Build history of the part. All positions in model axes, mm. A direction names the side the tool comes from. Round coordinates to 2 decimals unless told otherwise and drop trailing zeros. Write each loop counter-clockwise with the first axis right and the second up, starting at its lowest first coordinate (ties: lowest second). Pieces come first, ordered by that corner, then holes. Notation, with made-up numbers: (54, -0.75) - (94, -0.75) arc R15 cw to (94, 5.25) - close; hole circle Ø2 at (73.25, 6.25). An arc over 180 degrees is marked (long way). Answer as a JSON object with one key per item and string values. Group by question number.
Item 1: Slice it at D-D, the plane y = 112.5. List the corners of the cut face in (x, z), then the cut area to 3 significant figures.
Item 2: Slice it at C-C, the plane x = 0. Give the number of separate pieces and of enclosed holes in the cut face, then the cut area to 3 significant figures.
Item 3: Two-plate mould, pull along Z, no slides. Class faces 1 (the cylindrical face through (159.517, 16.224, 106.685)), 2 (the cylindrical face through (1.1, 16.22, -261.29)), 3 (the flat face through (158, 193, 91)), 4 (the cylindrical face through (-205.935, 208.776, 100.557)): +Z half, -Z half, draft (parallel to the pull), parting line (faces both ways), or undercut.
Item 4: Flat gauge pins, fed straight in: pin 1 (1.5 mm diameter, centred on y = 72.5, z = 44, fed in from -X); pin 2 (8 mm diameter, centred on y = 115, z = 98, fed in from +X); pin 3 (12 mm diameter, centred on x = 64.5, y = 72.5, fed in from +Z). Where does each tip first touch, or does it go through?
Item 5: Slice it at A-A, the plane z = -156. List the corners of the cut face in (x, y), then the cut area to 3 significant figures.
Item 6: Probe line 1 (X direction, y = 112, z = 120); line 2 (Z direction, x = 52, y = 96.5); line 3 (Z direction, x = -204, y = 197.5). List the from-to ranges inside material, lowest first. Write a range as from..to.
Item 7: Which spindle directions (+Z, -Z, +X, -X, +Y, -Y) get a long thin tool onto all of the face, cutting with end or side? Do faces 5 (the flat face through (122.633, 16.224, 128.537)), 6 (the cylindrical face through (94.619, 110.925, -103.186)), 7 (the cylindrical face through (55.179, 83.646, 152.605)). Say none if no direction does.
Item 8: Slice it at B-B, the plane y = 74.5. List the corners of the cut face in (x, z), then the cut area to 3 significant figures.
from build123d import *

# Parameters (mm, degrees)
SKETCH1_R                = 140
SKETCH1_R_2              = 97
BOSS_EXTRUDE3_DEPTH      = 225
BOSS_EXTRUDE4_START      = -32
SKETCH4_R                = 23.5
BOSS_EXTRUDE4_DEPTH      = 32
CIRPATTERN2_COUNT        = 3
MIRROR1_START            = -32
MIRROR1_COPY_1_SKETCH_R  = 23.5
MIRROR1_COPY_1_DEPTH     = 32
MIRROR1_COPY_2_SKETCH_R  = 23.5
MIRROR1_COPY_2_DEPTH     = 32
BOSS_EXTRUDE5_REACH      = 533.421
BOSS_EXTRUDE5_END_RADIUS = 140
SKETCH6_R                = 100
SKETCH7_R                = 50
CUT_EXTRUDE1_DEPTH       = 25
SKETCH8_R                = 28
CUT_EXTRUDE2_DEPTH       = 512.827938218
SKETCH9_R                = 12
CUT_EXTRUDE3_DEPTH       = 15
CIRPATTERN3_COUNT        = 3


with BuildPart() as part:
    # Sketch1 → Boss-Extrude3 (new body)
    with BuildSketch(Plane(origin=(0, 0, 0), x_dir=(1, 0, 0), z_dir=(0, 1, 0))):
        with Locations(Location((0, 0, 0), (0, 0, 270))):
            Circle(SKETCH1_R)
        with Locations(Location((0, 0, 0), (0, 0, 270))):
            Circle(SKETCH1_R_2, mode=Mode.SUBTRACT)
    extrude(amount=BOSS_EXTRUDE3_DEPTH)

    # Sketch4 → Boss-Extrude4 (add)
    with BuildSketch(Plane(origin=(0, 225, 0), x_dir=(1, 0, 0), z_dir=(0, 1, 0)).offset(BOSS_EXTRUDE4_START)):
        with BuildLine():
            ThreePointArc((50, 211.303564756), (0, 261.303564756), (-50, 211.303564756))
            Line((-50, 211.303564756), (-50, 130.766968306))
            ThreePointArc((-50, 130.766968306), (0, 140), (50, 130.766968306))
            Line((50, 130.766968306), (50, 211.303564756))
        make_face()
        with Locations(Location((0, 211.303564756, 0), (0, 0, 270))):
            Circle(SKETCH4_R, mode=Mode.SUBTRACT)
    boss_extrude4 = extrude(amount=BOSS_EXTRUDE4_DEPTH)

    # CirPattern2: Boss-Extrude4 ×3 about axis
    cirpattern2_axis = Axis((0, 0, 0), (0, 1, 0))
    for i in range(1, CIRPATTERN2_COUNT):
        add(boss_extrude4.rotate(cirpattern2_axis, i * 360 / CIRPATTERN2_COUNT))

    # Mirror1: Boss-Extrude4 across plane
    add(boss_extrude4.mirror(Plane.ZX.offset(112.5)))

    # Mirror1 copy 1 sketch → Mirror1 copy 1 (add)
    with BuildSketch(Plane(origin=(0, 0, 0), x_dir=(-0.4999999999999998, 0, -0.8660254037844387), z_dir=(0, -1, 0)).offset(MIRROR1_START)):
        with BuildLine():
            ThreePointArc((50, -211.303564756), (0, -261.303564756), (-50, -211.303564756))
            Line((-50, -211.303564756), (-50, -130.766968306))
            ThreePointArc((-50, -130.766968306), (0, -140), (50, -130.766968306))
            Line((50, -130.766968306), (50, -211.303564756))
        make_face()
        with Locations((0, -211.303564756)):
            Circle(MIRROR1_COPY_1_SKETCH_R, mode=Mode.SUBTRACT)
    extrude(amount=MIRROR1_COPY_1_DEPTH)

    # Mirror1 copy 2 sketch → Mirror1 copy 2 (add)
    with BuildSketch(Plane(origin=(0, 0, 0), x_dir=(-0.5000000000000004, 0, 0.8660254037844384), z_dir=(0, -1, 0)).offset(MIRROR1_START)):
        with BuildLine():
            ThreePointArc((50, -211.303564756), (0, -261.303564756), (-50, -211.303564756))
            Line((-50, -211.303564756), (-50, -130.766968306))
            ThreePointArc((-50, -130.766968306), (0, -140), (50, -130.766968306))
            Line((50, -130.766968306), (50, -211.303564756))
        make_face()
        with Locations((0, -211.303564756)):
            Circle(MIRROR1_COPY_2_SKETCH_R, mode=Mode.SUBTRACT)
    extrude(amount=MIRROR1_COPY_2_DEPTH)

    # Boss-Extrude5: up to this cylinder (the profile starts outside it)
    boss_extrude5_end = Plane(origin=(0, 112.5, 0), z_dir=(0, -1, 0)) * Cylinder(BOSS_EXTRUDE5_END_RADIUS, 1347.842, mode=Mode.PRIVATE)
    # Sketch6 → Boss-Extrude5 (add, up to the surface)
    with BuildSketch(Plane.XY.offset(160), mode=Mode.PRIVATE) as boss_extrude5_sk1:
        with Locations((0, 112.5)):
            Circle(SKETCH6_R)
    boss_extrude5_tool1 = extrude(boss_extrude5_sk1.sketch, amount=-BOSS_EXTRUDE5_REACH, mode=Mode.PRIVATE) - boss_extrude5_end
    add(boss_extrude5_tool1.solids().sort_by_distance((0, 112.5, 160))[0])

    # Sketch7 → Cut-Extrude1 (cut)
    with BuildSketch(Plane.XY.offset(160)):
        with Locations((0, 112.5)):
            Circle(SKETCH7_R)
    extrude(amount=-CUT_EXTRUDE1_DEPTH, mode=Mode.SUBTRACT)

    # Sketch8 → Cut-Extrude2 (cut, through all)
    with BuildSketch(Plane.XY.offset(135)):
        with Locations((0, 112.5)):
            Circle(SKETCH8_R)
    extrude(amount=-CUT_EXTRUDE2_DEPTH, mode=Mode.SUBTRACT)

    # Sketch9 → Cut-Extrude3 (cut)
    with BuildSketch(Plane.XY.offset(160)):
        with Locations((0, 186.428214738)):
            Circle(SKETCH9_R)
    cut_extrude3 = extrude(amount=-CUT_EXTRUDE3_DEPTH, mode=Mode.SUBTRACT)

    # CirPattern3: Cut-Extrude3 ×3 about axis
    cirpattern3_axis = Axis((0, 112.5, 0), (0, 0, 1))
    for i in range(1, CIRPATTERN3_COUNT):
        add(cut_extrude3.rotate(cirpattern3_axis, i * 360 / CIRPATTERN3_COUNT), mode=Mode.SUBTRACT)


solid = part.part
Geometry says:
{
 "1": {"outline": "(-100, 97.98) arc R140 ccw to (-28, -137.17) - (-28, -92.87) arc R97 cw to (-28, 92.87) - (-28, 135) - (-50, 135) - (-50, 160) - (-100, 160) - close; (28, -137.17) arc R140 ccw to (100, 97.98) - (100, 160) - (50, 160) - (50, 135) - (28, 135) - (28, 92.87) arc R97 cw to (28, -92.87) - close", "area": "31,500 mm^2"},
 "2": {"separate pieces": "6", "enclosed holes": "0", "area": "20,700 mm^2"},
 "3": {"face 1": "undercut", "face 2": "-Z half", "face 3": "draft", "face 4": "undercut"},
 "4": {"pin 1": "stops at x = -133.15", "pin 2": "stops at x = 103.75", "pin 3": "stops at z = 145"},
 "5": {"outline": "(-50, 0) - (50, 0) - (50, 32) - (-50, 32) - close; (-50, 193) - (50, 193) - (50, 225) - (-50, 225) - close", "area": "6,400 mm^2"},
 "6": {"line 1": "x = -100..-28, 28..100", "line 2": "z = -129.98..-81.88, 81.88..160", "line 3": "z = 60.04..95.12, 116.19..151.03"},
 "7": {"face 5": "+Z, -Y", "face 6": "none", "face 7": "+Z"},
 "8": {"outline": "(-92.5, 105.09) arc R140 ccw (long way) to (92.5, 105.09) - (92.5, 160) - (75.98, 160) - (75.98, 145) - (52.07, 145) - (52.07, 160) - (32.5, 160) - (32.5, 135) - (-32.5, 135) - (-32.5, 160) - (-52.07, 160) - (-52.07, 145) - (-75.98, 145) - (-75.98, 160) - (-92.5, 160) - close; hole circle Ø194 at (0, 0)", "area": "35,400 mm^2"}
}
